```python
from build123d import *

# Parameters (mm, degrees)
BOX_W          = 75
BOX_H          = 75
BOX_DEPTH      = 3
CYLINDER_R     = 10
CYLINDER_DEPTH = 3


with BuildPart() as part:
    # Box → Box (join)
    with BuildSketch(Plane.XY):
        with Locations((37.5, 37.5)):
            Rectangle(BOX_W, BOX_H)
    extrude(amount=BOX_DEPTH)

    # Cylinder → Cylinder (cut)
    with BuildSketch(Plane(origin=(37.5, 37.5, 0), x_dir=(0, -1, 0), z_dir=(0, 0, 1))):
        Circle(CYLINDER_R)
    extrude(amount=CYLINDER_DEPTH, mode=Mode.SUBTRACT)


solid = part.part
```
Work out the finished part from the listing and answer in its coordinate system (mm). Round coordinates to 2 decimals unless told otherwise and drop trailing zeros. Write each loop counter-clockwise with the first axis right and the second up, starting at its lowest first coordinate (ties: lowest second). Pieces come first, ordered by that corner, then holes.
1) Consider probe 1 along X at (y, z) = (37.5, 1.9); probe 2 along X at (y, z) = (31, 2.35); probe 3 along Y at (x, z) = (33, 2.7). Determine where each line is inside the solid, lowest interval first.
2) Determine the mould class of faces 1 (the face through (27.74, 39.67, 1.48)), 2 (the face through (0, 37, 1)), 3 (the face through (75, 37, 1)), 4 (the face through (29, 30, 3)) for opening direction X: pulls with the +X half, pulls with the -X half, needs draft (parallel to the pull), parting line crosses it, or undercut.
3) A cutting plane is placed at A-A on x = 37.5. Determine the outline of the cut face in (y, z).
4) A cutting plane is placed at C-C on z = 2.05. Determine the outline of the cut face in (x, y), and give its area (3 significant figures).
Entries:
1. probe 1: x = 0 to 27.5, 47.5 to 75
1. probe 2: x = 0 to 29.9, 45.1 to 75
1. probe 3: y = 0 to 28.57, 46.43 to 75
2. face 1: undercut
2. face 2: pulls with the -X half
2. face 3: pulls with the +X half
2. face 4: needs draft
3. outline: (0, 0) - (27.5, 0) - (27.5, 3) - (0, 3) - close; (47.5, 0) - (75, 0) - (75, 3) - (47.5, 3) - close
4. outline: (0, 0) - (75, 0) - (75, 75) - (0, 75) - close; hole circle Ø20 at (37.5, 37.5)
4. area: 5,310 mm2
